Input: part model. Units: mm. Frame: model coordinates. A direction names the side the tool comes from. Round coordinates to 2 decimals unless told otherwise and drop trailing zeros. Write each loop counter-clockwise with the first axis right and the second up, starting at its lowest first coordinate (ties: lowest second). Pieces come first, ordered by that corner, then holes. Notation, with made-up numbers: M -33,-24.75 L 18,-24.75 A24 ccw 18,-3.75 Z; hole C -30.75,50 d7. An arc over 180 degrees is marked long. Write each question's results on one line, items separated by ' | '. Start each with the question number.
```python
from build123d import *

# Parameters (mm, degrees)
F1_DEPTH  = 4
F2_T      = -1.8
F3_R      = 3.325
F3_R_2    = 2.2
F4_DEPTH  = 1.801
F3_R_3    = 1.6
F5_DEPTH  = 0.6
F3_R_4    = 5.675
F6_DEPTH  = 2.6
F3_R_5    = 2.5
F3_R_6    = 1.5
F7_DEPTH  = 3.6
F3_R_7    = 1.55
F8_DEPTH  = 3.9
F3_R_8    = 4
F9_DEPTH  = 6
F3_R_9    = 2.1
F10_DEPTH = 9.2


with BuildPart() as f1:
    # F0 (on Top) → F1 (new body)
    with BuildSketch(Plane.XY):
        with BuildLine():
            Line((-22.95, -42.3), (22.95, -42.3))
            ThreePointArc((22.95, -42.3), (28.2533008589, -40.1033008589), (30.45, -34.8))
            Line((30.45, -34.8), (30.45, 34.8))
            ThreePointArc((30.45, 34.8), (28.2533008589, 40.1033008589), (22.95, 42.3))
            Line((22.95, 42.3), (-22.95, 42.3))
            ThreePointArc((-22.95, 42.3), (-28.2533008589, 40.1033008589), (-30.45, 34.8))
            Line((-30.45, 34.8), (-30.45, -34.8))
            ThreePointArc((-30.45, -34.8), (-28.2533008589, -40.1033008589), (-22.95, -42.3))
        make_face()
    extrude(amount=F1_DEPTH)

    # F2
    f2_openings = [f1.faces().sort_by_distance(p)[0] for p in [
        (0, 0, 4),
    ]]
    offset(amount=F2_T, openings=f2_openings)

    # F3 (on face) → F4 (cut, through all)
    with BuildSketch(Plane.XY.offset(1.8)):
        with Locations((-21.22, 33.07)):
            Circle(F3_R)
        with Locations((-5.25, -1.2)):
            Circle(F3_R_2)
    extrude(amount=-F4_DEPTH, mode=Mode.SUBTRACT)

    # F3 (on face) → F5 (join)
    with BuildSketch(Plane.XY.offset(1.8)):
        with BuildLine():
            ThreePointArc((-4, 15.1), (0, 11.1), (4, 15.1))
            Line((4, 15.1), (4, 40.5))
            Line((4, 40.5), (-4, 40.5))
            Line((-4, 40.5), (-4, 15.1))
        make_face()
        with Locations((0, 13.1)):
            Circle(F3_R_3, mode=Mode.SUBTRACT)
    extrude(amount=F5_DEPTH)

    # F3 (on face) → F6 (join)
    with BuildSketch(Plane.XY.offset(1.8)):
        with Locations((-21.22, 33.07)):
            Circle(F3_R_4)
        with Locations((-21.22, 33.07)):
            Circle(F3_R, mode=Mode.SUBTRACT)
    extrude(amount=F6_DEPTH)

    # F3 (on face) → F7 (join)
    with BuildSketch(Plane.XY.offset(1.8)):
        with Locations((0, 13.1)):
            Circle(F3_R_3)
        with Locations((-24.35, 8.8)):
            Circle(F3_R_5)
        with Locations((-24.35, 8.8)):
            Circle(F3_R_6, mode=Mode.SUBTRACT)
    extrude(amount=F7_DEPTH)

    # F3 (on face) → F8 (join)
    with BuildSketch(Plane.XY.offset(1.8)):
        with Locations((10.85, -0.5)):
            Circle(F3_R_7)
    extrude(amount=F8_DEPTH)

    # F3 (on face) → F9 (join)
    with BuildSketch(Plane.XY.offset(1.8)):
        with Locations((-5.25, -1.2)):
            Circle(F3_R_8)
        with Locations((-5.25, -1.2)):
            Circle(F3_R_2, mode=Mode.SUBTRACT)
    extrude(amount=F9_DEPTH)

    # F3 (on face) → F10 (join)
    with BuildSketch(Plane.XY.offset(1.8)):
        with Locations((-12.15, 5)):
            Circle(F3_R_9)
    extrude(amount=F10_DEPTH)


solid = f1.part
```
1. Line query: L1, parallel to Y at x = 11, z = 3.25; L2, parallel to Y at x = 5.5, z = 3.75; L3, parallel to Y at x = -5.5, z = 1.5. Output: solid intervals per line, ascending. Write a range as from..to.
2. Access query for faces 1 (the face through (-5.771, 2.766, 4.758)), 2 (the face through (11, 0, 5.7)), 3 (the face through (28.195, -40.161, 1.972)). Directions: +Z, -Z, +X, -X, +Y, -Y. A direction counts if a zero-diameter tool reaches every point of the face in a straight line with its end or side. Return the directions, or none.
3. Cut plane A-A on y = 5. Output: boundary loops of the cut face in (x, z).
4. Cut plane B-B on x = -5.25. Output: boundary loops of the cut face in (y, z).
5. Cut plane D-D on z = 9.5. Output: boundary loops of the cut face in (x, y).
6. Draft query along X for faces 4 (the face through (-30.45, 0, 2)), 5 (the face through (0, 40.5, 3)), 6 (the face through (-27.02, -38.79, 2.88)), 7 (the face through (-24, 7, 5.4)). Return one class per face: +X half, -X half, draft (parallel to the pull), parting line (faces both ways), or undercut.
7. Cut plane C-C on x = 15.5. Output: boundary loops of the cut face in (y, z).
8. Contact query for flat-ended pins moving along their axis: P1, Ø5, axis at x = -24.35, y = 8.8, coming from the +Z side; P2, Ø2.5, axis at x = -5.25, y = -1.2, coming from the -Z side; P3, Ø2, axis at x = 12, z = 5.5, coming from the +Y side; P4, Ø9, axis at x = -21.5, y = 34.5, coming from the +Z side. Output: stop coordinate, or through.
Answers follow:
1) L1: y = -42.3..-40.5, -2.04..1.04, 40.5..42.3 | L2: y = -42.3..-40.5, 40.5..42.3 | L3: y = -42.3..-3.39, 0.99..42.3
2) face 1: +Z | face 2: +Z, +X, +Y, -Y | face 3: +Z, -Z, +X, -Y
3) outline: M -30.45,0 L 30.45,0 L 30.45,4 L 28.65,4 L 28.65,1.8 L -10.05,1.8 L -10.05,11 L -14.25,11 L -14.25,1.8 L -28.65,1.8 L -28.65,4 L -30.45,4 Z
4) outline: M -42.3,0 L -3.4,0 L -3.4,7.8 L -5.2,7.8 L -5.2,1.8 L -40.5,1.8 L -40.5,4 L -42.3,4 Z; M 1,0 L 42.3,0 L 42.3,4 L 40.5,4 L 40.5,1.8 L 2.8,1.8 L 2.8,7.8 L 1,7.8 Z
5) outline: C -12.15,5 d4.2
6) face 4: -X half | face 5: undercut | face 6: undercut | face 7: draft
7) outline: M -42.3,0 L 42.3,0 L 42.3,4 L 40.5,4 L 40.5,1.8 L -40.5,1.8 L -40.5,4 L -42.3,4 Z
8) P1: stops at z = 5.4 | P2: passes through | P3: stops at y = 1.04 | P4: stops at z = 4.4
